Could you check a few things on this drawing? It's one solid part, dimensions in mm from its lowest x, y, z. A direction names the side the tool comes from. Give positions to 0.01 mm unless a question says otherwise; leave off trailing zeros.
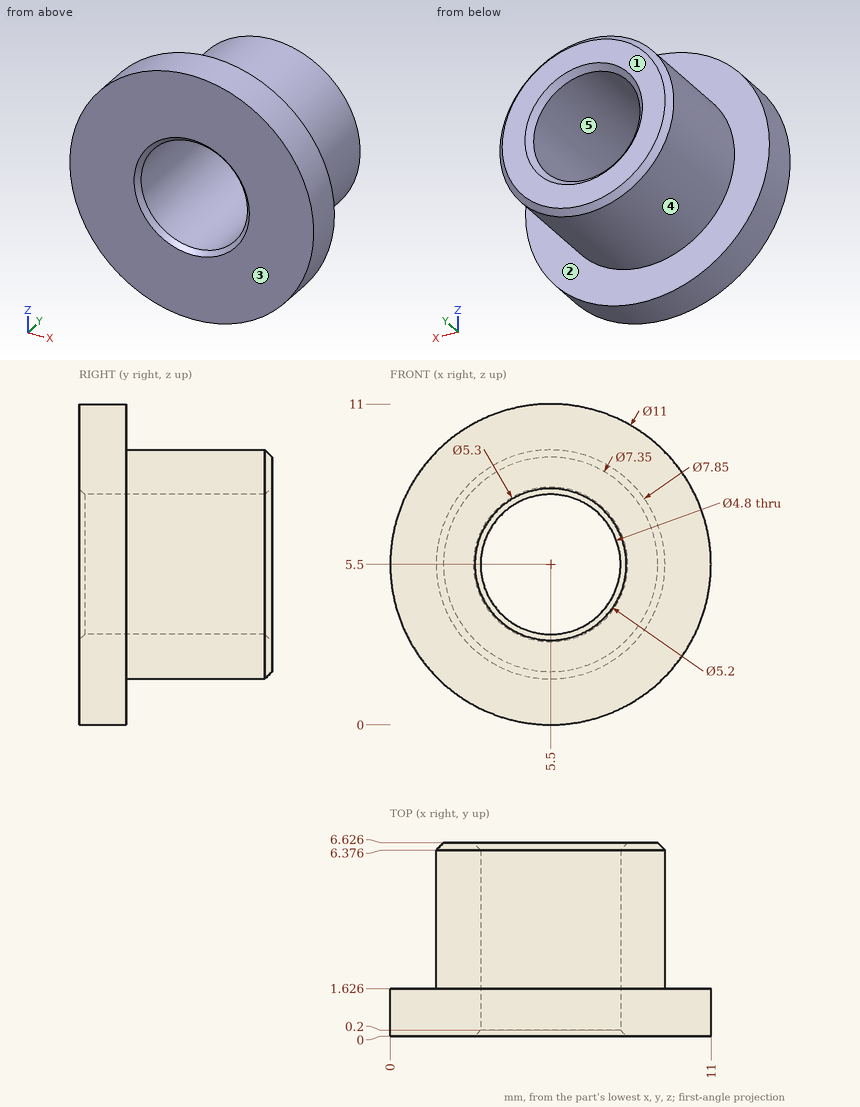
Q1. I'm going to push flat-ended pins straight in: P1, Ø1.5, axis at x = 1.5, y = 5.5, coming from the +Z side; P2, Ø1, axis at y = 2, z = 3.5, coming from the +X side; P3, Ø3, axis at x = 7.5, y = 5.5, coming from the +Z side; P4, Ø4, axis at x = 5.5, z = 5.5, coming from the +Y side. Where does each tip first touch, or does it pass through?
Filled sheet:
P1: stops at z = 7.7
P2: stops at x = 10.74
P3: stops at z = 9.39
P4: passes through
Q2. Thinking about a two-plate mould opening in X: for the marked faces 3, 4 and 5, which applies, released by +X, released by -X, zero draft, split by the parting line, or undercut?
Filled sheet:
face 3: zero draft
face 4: split by the parting line
face 5: undercut
Q3. For the marked faces 1 and 2, which set-ups out of +Z, -Z, +X, -X, +Y, -Y let a thin tool reach every point of the face, with its end or its side?
Filled sheet:
face 1: +Z, -Z, +X, -X, +Y
face 2: +Y
Q4. I need wall thicknesses on L1, parallel to Z at x = 5.5, y = 4.25 (1 decimal); L2, parallel to X at y = 4.5, z = 4.5 (1 decimal); L3, parallel to Y at x = 1.5, z = 5.75 (1 decimal). Which ranges of each line are inside material? Lowest first, please.
Filled sheet:
L1: z = 1.6 to 3.1, 7.9 to 9.4
L2: x = 1.7 to 3.3, 7.7 to 9.3
L3: y = 0 to 1.6
